Input: part model. Units: mm. Frame: model coordinates. Face numbers are marked on the shaded views. A direction names the side the tool comes from. Coordinates: 2 decimals unless noted, no trailing zeros. Order: outer loops, then holes, each group sorted by start corner. A loop starts at its lowest first (then second) coordinate and runs counter-clockwise, first axis right, second up. Notation, with made-up numbers: (-33.5, 36) -> (23.5, 36) arc R22 ccw to (23.5, 57) -> close; hole circle Ø2 at (66, 14). An arc over 180 degrees is marked (long way). Answer as CSV lines item,"result".
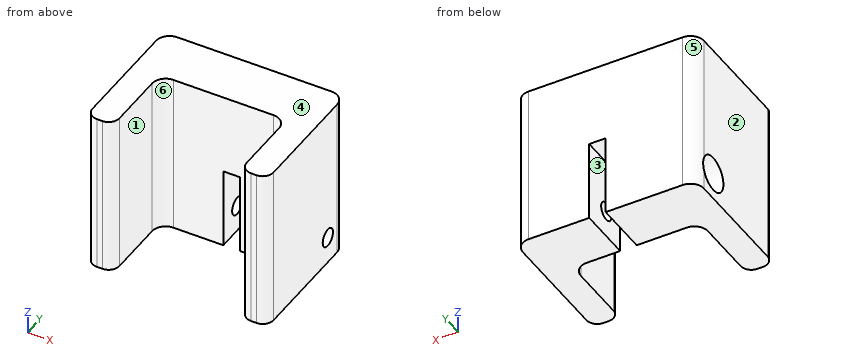
from build123d import *

# Parameters (mm, degrees)
F1_DEPTH       = 30
F2_W           = 3.0429003396
F2_H           = 15
F3_DEPTH       = 25.001
F5_D           = 3.3
F5_START       = 0.0125315
F5_CBORE_D     = 6.5
F5_CBORE_DEPTH = 3


with BuildPart() as f1:
    # F0 (on Top) → F1 (new body)
    with BuildSketch(Plane.XY):
        with BuildLine():
            ThreePointArc((-11.2567170643, -9.8372937679), (-10.6709306267, -11.2515073303), (-9.2567170643, -11.8372937679))
            Line((-9.2567170643, -11.8372937679), (-8.2567170643, -11.8372937679))
            ThreePointArc((-8.2567170643, -11.8372937679), (-6.8425035019, -11.2515073303), (-6.2567170643, -9.8372937679))
            Line((-6.2567170643, -9.8372937679), (-6.2567170643, 0.6627062321))
            ThreePointArc((-6.2567170643, 0.6627062321), (-5.5244840173, 2.430473185), (-3.7567170643, 3.1627062321))
            Line((-3.7567170643, 3.1627062321), (14.7432829357, 3.1627062321))
            ThreePointArc((14.7432829357, 3.1627062321), (16.5110498887, 2.430473185), (17.2432829357, 0.6627062321))
            Line((17.2432829357, 0.6627062321), (17.2432829357, -9.8372937679))
            ThreePointArc((17.2432829357, -9.8372937679), (17.8290693733, -11.2515073303), (19.2432829357, -11.8372937679))
            Line((19.2432829357, -11.8372937679), (20.2432829357, -11.8372937679))
            ThreePointArc((20.2432829357, -11.8372937679), (21.6574964981, -11.2515073303), (22.2432829357, -9.8372937679))
            Line((22.2432829357, -9.8372937679), (22.2432829357, 10.6627062321))
            ThreePointArc((22.2432829357, 10.6627062321), (21.5110498887, 12.430473185), (19.7432829357, 13.1627062321))
            Line((19.7432829357, 13.1627062321), (-8.7567170643, 13.1627062321))
            ThreePointArc((-8.7567170643, 13.1627062321), (-10.5244840173, 12.430473185), (-11.2567170643, 10.6627062321))
            Line((-11.2567170643, 10.6627062321), (-11.2567170643, -9.8372937679))
        make_face()
    extrude(amount=F1_DEPTH)

    # F2 (on face) → F3 (cut, through all)
    with BuildSketch(Plane(origin=(0, 13.1627062321, 0), x_dir=(-1, 0, 0), z_dir=(0, 1, 0))):
        with Locations((-7.0147331055, 7.5)):
            Rectangle(F2_W, F2_H)
    extrude(amount=-F3_DEPTH, mode=Mode.SUBTRACT)

    # F5 (through all)
    # its depths count from where the whole tool has entered the part; down to there all is cleared
    with Locations(Plane(origin=(-11.2567170643, 0, 0), x_dir=(0, -1, 0), z_dir=(-1, 0, 0)).offset(-F5_START)):
        with Locations((-7.6627062321, 5)):
            CounterBoreHole(F5_D / 2, F5_CBORE_D / 2, F5_CBORE_DEPTH)


solid = f1.part
1. Cut plane D-D (z = 26). Return the cut outline in (x, y).
Findings:
outline,"(-11.26, -9.84) arc R2 ccw to (-9.26, -11.84) -> (-8.26, -11.84) arc R2 ccw to (-6.26, -9.84) -> (-6.26, 0.66) arc R2.5 cw to (-3.76, 3.16) -> (14.74, 3.16) arc R2.5 cw to (17.24, 0.66) -> (17.24, -9.84) arc R2 ccw to (19.24, -11.84) -> (20.24, -11.84) arc R2 ccw to (22.24, -9.84) -> (22.24, 10.66) arc R2.5 ccw to (19.74, 13.16) -> (-8.76, 13.16) arc R2.5 ccw to (-11.26, 10.66) -> close"
2. Reachability of the marked faces 1, 2 and 3 from +Z, -Z, +X, -X, +Y, -Y: full face, straight path, thin tool, end or side. Return the list, or none.
Findings:
face 1,"+Z, -Z, -Y"
face 2,"+Z, -Z, -X, +Y, -Y"
face 3,"-Z, +Y, -Y"
3. Contact query for flat-ended pins moving along their axis: pin 1 (3 mm diameter, centred on y = 9, z = 5, fed in from -X); pin 2 (1.5 mm diameter, centred on x = 7.5, z = 13.5, fed in from +Y); pin 3 (12 mm diameter, centred on x = 3, z = 19, fed in from -Y); pin 4 (12 mm diameter, centred on x = 0, z = 19, fed in from -Y). Output: stop coordinate, or through.
Findings:
pin 1,"stops at x = -8.24"
pin 2,"passes through"
pin 3,"stops at y = 3.16"
pin 4,"stops at y = 1.77"
4. Cut plane C-C (x = -2). Return the cut outline in (y, z).
Findings:
outline,"(3.16, 0) -> (13.16, 0) -> (13.16, 30) -> (3.16, 30) -> close; hole circle Ø3.3 at (7.66, 5)"
5. Cut plane A-A (z = 14). Return the cut outline in (x, y).
Findings:
outline,"(-11.26, -9.84) arc R2 ccw to (-9.26, -11.84) -> (-8.26, -11.84) arc R2 ccw to (-6.26, -9.84) -> (-6.26, 0.66) arc R2.5 cw to (-3.76, 3.16) -> (5.49, 3.16) -> (5.49, 13.16) -> (-8.76, 13.16) arc R2.5 ccw to (-11.26, 10.66) -> close; (8.54, 3.16) -> (14.74, 3.16) arc R2.5 cw to (17.24, 0.66) -> (17.24, -9.84) arc R2 ccw to (19.24, -11.84) -> (20.24, -11.84) arc R2 ccw to (22.24, -9.84) -> (22.24, 10.66) arc R2.5 ccw to (19.74, 13.16) -> (8.54, 13.16) -> close"
6. Cut plane B-B (z = 5). State how many separate pieces and enclosed holes the cut face has, plus the area to 3 significant figures.
Findings:
separate pieces,"4"
enclosed holes,"0"
area,"341 mm2"
7. Ray query, line 1 along X through (y, z) = (-6.75, 28); line 2 along X through (y, z) = (6, 6); line 3 along Y through (x, z) = (0, 25.5). Return the intervals inside material, ascending.
Findings:
line 1,"x = -11.26 to -6.26, 17.24 to 22.24"
line 2,"x = -8.24 to 5.49, 8.54 to 22.24"
line 3,"y = 3.16 to 13.16"
8. Mould query, pull axis X, two halves, no side actions, for the marked faces 4, 5 and 6. Classes: released by +X, released by -X, zero draft, split by the parting line, or undercut.
Findings:
face 4,"zero draft"
face 5,"released by -X"
face 6,"undercut"
